```python
from build123d import *

# Parameters (mm, degrees)
CROQUIS1_R              = 1.5
CROQUIS1_W              = 6.1
CROQUIS1_H              = 25
CROQUIS1_H_2            = 15
CROQUIS1_R_2            = 2
CROQUIS1_R_3            = 6.75
CROQUIS1_R_4            = 5.25
SALIENTE_EXTRUIR1_DEPTH = 6


with BuildPart() as part:
    # Croquis1 → Saliente-Extruir1 (new body)
    with BuildSketch(Plane.XY):
        with BuildLine():
            Line((87.635637669, 16), (32.115377174, 16))
            ThreePointArc((32.115377174, 16), (30.701163612, 15.414213562), (30.115377174, 14))
            Line((30.115377174, 14), (30.115377174, 10.910010016))
            Line((30.115377174, 10.910010016), (-30.115377174, 10.910010016))
            Line((-30.115377174, 10.910010016), (-30.115377174, 14))
            ThreePointArc((-30.115377174, 14), (-30.701163612, 15.414213562), (-32.115377174, 16))
            Line((-32.115377174, 16), (-44.664398505, 16))
            Line((-44.664398505, 16), (-87.635637669, 16))
            Line((-87.635637669, 16), (-109, 16))
            ThreePointArc((-109, 16), (-110.414213562, 15.414213562), (-111, 14))
            Line((-111, 14), (-111, 0))
            Line((-111, 0), (-111, -15.999955929))
            ThreePointArc((-111, -15.999955929), (-114.684754838, -37.224148725), (-127.277573278, -54.701697231))
            Line((-127.277573278, -54.701697231), (-135.277573278, -54.701697231))
            Line((-135.277573278, -54.701697231), (-140.277573278, -54.701697231))
            ThreePointArc((-140.277573278, -54.701697231), (-148.762854653, -58.216415857), (-152.277573278, -66.701697231))
            Line((-152.277573278, -66.701697231), (-152.277573278, -303.912438798))
            ThreePointArc((-152.277573278, -303.912438798), (-148.762854653, -312.397720172), (-140.277573278, -315.912438798))
            Line((-140.277573278, -315.912438798), (-135.277573278, -315.912438798))
            Line((-135.277573278, -315.912438798), (-119.364295205, -315.912438798))
            Line((-119.364295205, -315.912438798), (119.364429455, -315.912438798))
            Line((119.364429455, -315.912438798), (130.295105026, -315.912438798))
            Line((130.295105026, -315.912438798), (146.942872896, -315.912438798))
            ThreePointArc((146.942872896, -315.912438798), (155.42815427, -312.397720172), (158.942872896, -303.912438798))
            Line((158.942872896, -303.912438798), (158.942872896, -70.770984471))
            Line((158.942872896, -70.770984471), (158.942872896, -66.701697231))
            ThreePointArc((158.942872896, -66.701697231), (155.42815427, -58.216415857), (146.942872896, -54.701697231))
            Line((146.942872896, -54.701697231), (126.134028278, -54.701697231))
            ThreePointArc((126.134028278, -54.701697231), (114.918041875, -36.777730062), (111, -15.999955929))
            Line((111, -15.999955929), (111, 14))
            ThreePointArc((111, 14), (110.414213562, 15.414213562), (109, 16))
            Line((109, 16), (87.635637669, 16))
        make_face()
        with Locations((-138.277573278, -305.912438798)):
            Circle(CROQUIS1_R, mode=Mode.SUBTRACT)
        with Locations((-95, -282.201697231)):
            Rectangle(CROQUIS1_W, CROQUIS1_H, mode=Mode.SUBTRACT)
        with Locations((-95, -239.701697231)):
            Circle(CROQUIS1_R, mode=Mode.SUBTRACT)
        Polygon((-3.049885808, -294.789219369), (-3.049896429, -269.789219369), (3.050103571, -269.789216778), (3.050114192, -294.789216778), align=None, mode=Mode.SUBTRACT)
        with Locations((9.0826e-05, -239.789218073)):
            Circle(CROQUIS1_R, mode=Mode.SUBTRACT)
        with Locations((-95, -197.201697231)):
            Rectangle(CROQUIS1_W, CROQUIS1_H, mode=Mode.SUBTRACT)
        with Locations((-95, -154.701697231)):
            Circle(CROQUIS1_R, mode=Mode.SUBTRACT)
        Polygon((-3.049921919, -209.789219369), (-3.04993254, -184.789219369), (3.05006746, -184.789216778), (3.050078081, -209.789216778), align=None, mode=Mode.SUBTRACT)
        with Locations((5.4715e-05, -154.789218073)):
            Circle(CROQUIS1_R, mode=Mode.SUBTRACT)
        Polygon((91.950125201, -294.701658167), (91.95011458, -269.701658167), (98.05011458, -269.701655576), (98.050125201, -294.701655576), align=None, mode=Mode.SUBTRACT)
        with Locations((146.722426722, -305.912438798)):
            Circle(CROQUIS1_R, mode=Mode.SUBTRACT)
        with Locations((95.000101835, -239.701656871)):
            Circle(CROQUIS1_R, mode=Mode.SUBTRACT)
        Polygon((91.95008909, -209.701658167), (91.950078469, -184.701658167), (98.050078469, -184.701655576), (98.05008909, -209.701655576), align=None, mode=Mode.SUBTRACT)
        with Locations((95.000065724, -154.701656871)):
            Circle(CROQUIS1_R, mode=Mode.SUBTRACT)
        with Locations((-95, -112.201697231)):
            Rectangle(CROQUIS1_W, CROQUIS1_H, mode=Mode.SUBTRACT)
        with Locations((-95, -69.701697231)):
            Circle(CROQUIS1_R, mode=Mode.SUBTRACT)
        Polygon((-3.04995803, -124.789219369), (-3.049968651, -99.789219369), (3.050031349, -99.789216778), (3.05004197, -124.789216778), align=None, mode=Mode.SUBTRACT)
        with Locations((1.8603e-05, -69.789218073)):
            Circle(CROQUIS1_R, mode=Mode.SUBTRACT)
        with Locations((-138.277573278, -60.912438798)):
            Circle(CROQUIS1_R, mode=Mode.SUBTRACT)
        with Locations((-95, -41.5)):
            Rectangle(CROQUIS1_W, CROQUIS1_H_2, mode=Mode.SUBTRACT)
        with Locations((-95, -26)):
            Circle(CROQUIS1_R, mode=Mode.SUBTRACT)
        with Locations((-106.313708499, -11.313708499)):
            Circle(CROQUIS1_R_2, mode=Mode.SUBTRACT)
        with Locations((-83.686291501, -11.313708499)):
            Circle(CROQUIS1_R_2, mode=Mode.SUBTRACT)
        with Locations((-95, 0)):
            Circle(CROQUIS1_R_3, mode=Mode.SUBTRACT)
        with Locations((-106.313708499, 11.313708499)):
            Circle(CROQUIS1_R_2, mode=Mode.SUBTRACT)
        with Locations((-83.686291501, 11.313708499)):
            Circle(CROQUIS1_R_2, mode=Mode.SUBTRACT)
        Polygon((-3.049990229, -48.999960936), (-3.049996601, -33.999960936), (3.050003399, -33.999958344), (3.050009771, -48.999958344), align=None, mode=Mode.SUBTRACT)
        with Locations((0.004600085, -25.999981675)):
            Circle(CROQUIS1_R, mode=Mode.SUBTRACT)
        with Locations((-5.656854249, -5.656854249)):
            Circle(CROQUIS1_R, mode=Mode.SUBTRACT)
        Circle(CROQUIS1_R_4, mode=Mode.SUBTRACT)
        with Locations((-5.656854249, 5.656854249)):
            Circle(CROQUIS1_R, mode=Mode.SUBTRACT)
        Polygon((91.950052978, -124.701658167), (91.950042357, -99.701658167), (98.050042357, -99.701655576), (98.050052978, -124.701655576), align=None, mode=Mode.SUBTRACT)
        with Locations((95.000029612, -69.701656871)):
            Circle(CROQUIS1_R, mode=Mode.SUBTRACT)
        with Locations((5.656854249, -5.656854249)):
            Circle(CROQUIS1_R, mode=Mode.SUBTRACT)
        with Locations((5.656854249, 5.656854249)):
            Circle(CROQUIS1_R, mode=Mode.SUBTRACT)
        Polygon((91.950020817, -48.999960936), (91.950014445, -33.999960936), (98.050014445, -33.999958344), (98.050020817, -48.999958344), align=None, mode=Mode.SUBTRACT)
        with Locations((95.000011046, -25.99995964)):
            Circle(CROQUIS1_R, mode=Mode.SUBTRACT)
        with Locations((146.722426722, -60.912438798)):
            Circle(CROQUIS1_R, mode=Mode.SUBTRACT)
        with Locations((83.686291501, -11.313708499)):
            Circle(CROQUIS1_R_2, mode=Mode.SUBTRACT)
        with Locations((106.313708499, -11.313708499)):
            Circle(CROQUIS1_R_2, mode=Mode.SUBTRACT)
        with Locations((95, 0)):
            Circle(CROQUIS1_R_3, mode=Mode.SUBTRACT)
        with Locations((83.686291501, 11.313708499)):
            Circle(CROQUIS1_R_2, mode=Mode.SUBTRACT)
        with Locations((106.313708499, 11.313708499)):
            Circle(CROQUIS1_R_2, mode=Mode.SUBTRACT)
    extrude(amount=SALIENTE_EXTRUIR1_DEPTH)


solid = part.part
```
Could you check a few things on this model? Use its own coordinates, in mm. Round coordinates to 2 decimals unless told otherwise and drop trailing zeros. Loops run counter-clockwise (first coordinate to the right, second up) from the corner with the lowest first, then second, coordinate; pieces in that order, holes last. Notation, with made-up numbers: (17.5, 48) - (29.5, 48) arc R17 cw to (29.5, 71) - close; hole circle Ø6 at (-37.5, 34). An arc over 180 degrees is marked (long way). Use CSV: the item, a comma, the result in double quotes.
Item 1: If we section it at C-C on z = 2.9: Count the separate pieces of the cut face and the enclosed holes in it, then the cut area to 3 significant figures.
Here are the results:
separate pieces,"1"
enclosed holes,"43"
area,"94,700 mm²"
Item 2: Will these pins go through, and if not, where does the flat tip stop? pin 1 (5 mm diameter, centred on x = 0, y = -69.79, fed in from +Z); pin 2 (1.8 mm diameter, centred on y = -39.5, z = 3, fed in from +X); pin 3 (2.5 mm diameter, centred on x = 95, y = -239.7, fed in from -Z); pin 4 (1.5 mm diameter, centred on y = 12.5, z = 4, fed in from +X).
Here are the results:
pin 1,"stops at z = 6"
pin 2,"stops at x = 116.48"
pin 3,"passes through"
pin 4,"stops at x = 111"
Item 3: If we mould it in two halves opening along Y, with no side actions, what happens to faces 1 (the flat face through (1, -148, 0)), 2 (the cylindrical face through (5, 1.6, 3)), 3 (the cylindrical face through (-148.669, -58.124, 2.958))? For each: pulls with the +Y half, pulls with the -Y half, needs draft (parallel to the pull), parting line crosses it, or undercut.
Here are the results:
face 1,"needs draft"
face 2,"undercut"
face 3,"pulls with the +Y half"
Item 4: I need wall thicknesses on L1, parallel to X at y = -199, z = 1.55; L2, parallel to X at y = -45.5, z = 4.95; L3, parallel to Y at x = 82, z = 0.7. Which ranges of each line are inside material? Lowest first, please. Write a range as [from, to].
Here are the results:
L1,"x = [-152.28, -98.05], [-91.95, -3.05], [3.05, 91.95], [98.05, 158.94]"
L2,"x = [-119.17, -98.05], [-91.95, -3.05], [3.05, 91.95], [98.05, 119.22]"
L3,"y = [-315.91, -12.39], [-10.24, 10.24], [12.39, 16]"
Item 5: If we section it at B-B on x = -22: List the corners of the cut face in (y, z) for me, then the cut area to 3 significant figures.
Here are the results:
outline,"(-315.91, 0) - (10.91, 0) - (10.91, 6) - (-315.91, 6) - close"
area,"1,960 mm²"
Item 6: If we section it at A-A on y = 0: List the corners of the cut face in (x, z) for me.
Here are the results:
outline,"(-111, 0) - (-101.75, 0) - (-101.75, 6) - (-111, 6) - close; (-88.25, 0) - (-5.25, 0) - (-5.25, 6) - (-88.25, 6) - close; (5.25, 0) - (88.25, 0) - (88.25, 6) - (5.25, 6) - close; (101.75, 0) - (111, 0) - (111, 6) - (101.75, 6) - close"
